```python
from build123d import *

# Parameters (mm, degrees)
ESQUISSE1_R             = 1.5
EXTRUSION1_DEPTH        = 5
ESQUISSE2_W             = 45
ESQUISSE2_H             = 5
EXTRUSION2_DEPTH        = 95
EXTRUSION3_DEPTH        = 5
ESQUISSE4_W             = 95
ESQUISSE4_H             = 50
EXTRUSION4_DEPTH        = 5
ESQUISSE5_W             = 100
ESQUISSE5_H             = 5
EXTRUSION5_DEPTH        = 40
ESQUISSE6_W             = 40
ESQUISSE6_H             = 50
EXTRUSION6_DEPTH        = 5
EXTRUSION7_DEPTH        = 5
ENL_V_MAT_EXTRU_1_REACH = 102
ESQUISSE8_R             = 1.5
ENL_V_MAT_EXTRU_2_REACH = 7
ESQUISSE9_R             = 1.5
BOSS_EXTRU_1_DEPTH      = 5
BOSS_EXTRU_2_DEPTH      = 5
ESQUISSE16_R            = 1.5
ENL_V_MAT_EXTRU_3_DEPTH = 4


with BuildPart() as part:
    # Esquisse1 → Extrusion1 (new body)
    with BuildSketch(Plane.XY):
        Polygon((0, 0), (45, 0), (45, 45), (45, 55), (0, 55), (0, 45), align=None)
        with Locations((31.692388155, 31.692388155)):
            Circle(ESQUISSE1_R, mode=Mode.SUBTRACT)
        with Locations((31.692388155, 13.307611845)):
            Circle(ESQUISSE1_R, mode=Mode.SUBTRACT)
        with Locations((13.307611845, 13.307611845)):
            Circle(ESQUISSE1_R, mode=Mode.SUBTRACT)
        with Locations((13.307611845, 31.692388155)):
            Circle(ESQUISSE1_R, mode=Mode.SUBTRACT)
        with BuildLine():
            Line((13.5, 26.858898944), (13.5, 18.141101056))
            ThreePointArc((13.5, 18.141101056), (22.5, 12.5), (31.5, 18.141101056))
            Line((31.5, 18.141101056), (31.5, 26.858898944))
            ThreePointArc((31.5, 26.858898944), (22.5, 32.5), (13.5, 26.858898944))
        make_face(mode=Mode.SUBTRACT)
    extrude(amount=EXTRUSION1_DEPTH)

    # Esquisse2 → Extrusion2 (add)
    with BuildSketch(Plane.XY.offset(5)):
        with Locations((22.5, 2.5)):
            Rectangle(ESQUISSE2_W, ESQUISSE2_H)
    extrude(amount=EXTRUSION2_DEPTH)

    # Esquisse3 → Extrusion3 (add)
    with BuildSketch(Plane(origin=(45, 0, 0), x_dir=(0, 0, -1), z_dir=(1, 0, 0))):
        Polygon((-5, 5), (-5, 55), (-25, 55), (-25, 50), (-55, 5), align=None)
    extrude(amount=-EXTRUSION3_DEPTH)

    # Esquisse4 → Extrusion4 (add)
    with BuildSketch(Plane.ZY):
        with Locations((52.5, 30)):
            Rectangle(ESQUISSE4_W, ESQUISSE4_H)
    extrude(amount=-EXTRUSION4_DEPTH)

    # Esquisse5 → Extrusion5 (add)
    with BuildSketch(Plane.ZY):
        with Locations((50, 2.5)):
            Rectangle(ESQUISSE5_W, ESQUISSE5_H)
    extrude(amount=EXTRUSION5_DEPTH)

    # Esquisse6 → Extrusion6 (add)
    with BuildSketch(Plane.XY.offset(100)):
        with Locations((-20, 30)):
            Rectangle(ESQUISSE6_W, ESQUISSE6_H)
    extrude(amount=-EXTRUSION6_DEPTH)

    # Esquisse7 → Extrusion7 (add)
    with BuildSketch(Plane.ZY.offset(40)):
        Polygon((95, 5), (95, 55), (75, 55), (75, 50), (45, 5), align=None)
    extrude(amount=-EXTRUSION7_DEPTH)

    # Esquisse8 → Enlèv. mat.-Extru.1 (cut, up to next)
    with BuildSketch(Plane.XY.offset(100), mode=Mode.PRIVATE) as enl_v_mat_extru_1_sk1:
        with Locations((-8.307611845, 13.307611845)):
            Circle(ESQUISSE8_R)
    enl_v_mat_extru_1_tool1 = extrude(enl_v_mat_extru_1_sk1.sketch, amount=-ENL_V_MAT_EXTRU_1_REACH, mode=Mode.PRIVATE) & part.part
    add(enl_v_mat_extru_1_tool1.solids().sort_by_distance((-8.307612, 13.307612, 100))[0], mode=Mode.SUBTRACT)
    # Esquisse8 → Enlèv. mat.-Extru.1 (cut, up to next)
    with BuildSketch(Plane.XY.offset(100), mode=Mode.PRIVATE) as enl_v_mat_extru_1_sk2:
        with Locations((-8.307611845, 31.692388155)):
            Circle(ESQUISSE8_R)
    enl_v_mat_extru_1_tool2 = extrude(enl_v_mat_extru_1_sk2.sketch, amount=-ENL_V_MAT_EXTRU_1_REACH, mode=Mode.PRIVATE) & part.part
    add(enl_v_mat_extru_1_tool2.solids().sort_by_distance((-8.307612, 31.692388, 100))[0], mode=Mode.SUBTRACT)
    # Esquisse8 → Enlèv. mat.-Extru.1 (cut, up to next)
    with BuildSketch(Plane.XY.offset(100), mode=Mode.PRIVATE) as enl_v_mat_extru_1_sk3:
        with Locations((-26.692388155, 31.692388155)):
            Circle(ESQUISSE8_R)
    enl_v_mat_extru_1_tool3 = extrude(enl_v_mat_extru_1_sk3.sketch, amount=-ENL_V_MAT_EXTRU_1_REACH, mode=Mode.PRIVATE) & part.part
    add(enl_v_mat_extru_1_tool3.solids().sort_by_distance((-26.692388, 31.692388, 100))[0], mode=Mode.SUBTRACT)
    # Esquisse8 → Enlèv. mat.-Extru.1 (cut, up to next)
    with BuildSketch(Plane.XY.offset(100), mode=Mode.PRIVATE) as enl_v_mat_extru_1_sk4:
        with Locations((-26.692388155, 13.307611845)):
            Circle(ESQUISSE8_R)
    enl_v_mat_extru_1_tool4 = extrude(enl_v_mat_extru_1_sk4.sketch, amount=-ENL_V_MAT_EXTRU_1_REACH, mode=Mode.PRIVATE) & part.part
    add(enl_v_mat_extru_1_tool4.solids().sort_by_distance((-26.692388, 13.307612, 100))[0], mode=Mode.SUBTRACT)
    # Esquisse8 → Enlèv. mat.-Extru.1 (cut, up to next)
    with BuildSketch(Plane.XY.offset(100), mode=Mode.PRIVATE) as enl_v_mat_extru_1_sk5:
        with BuildLine():
            Line((-26.5, 18.141101056), (-26.5, 26.858898944))
            ThreePointArc((-26.5, 26.858898944), (-17.5, 32.5), (-8.5, 26.858898944))
            Line((-8.5, 26.858898944), (-8.5, 18.141101056))
            ThreePointArc((-8.5, 18.141101056), (-17.5, 12.5), (-26.5, 18.141101056))
        make_face()
    enl_v_mat_extru_1_tool5 = extrude(enl_v_mat_extru_1_sk5.sketch, amount=-ENL_V_MAT_EXTRU_1_REACH, mode=Mode.PRIVATE) & part.part
    add(enl_v_mat_extru_1_tool5.solids().sort_by_distance((-17.5, 22.5, 100))[0], mode=Mode.SUBTRACT)

    # Esquisse9 → Enlèv. mat.-Extru.2 (cut, up to next)
    with BuildSketch(Plane(origin=(0, 5, 0), x_dir=(-1, 0, 0), z_dir=(0, 1, 0)), mode=Mode.PRIVATE) as enl_v_mat_extru_2_sk1:
        with Locations((-40, 95)):
            Circle(ESQUISSE9_R)
    enl_v_mat_extru_2_tool1 = extrude(enl_v_mat_extru_2_sk1.sketch, amount=-ENL_V_MAT_EXTRU_2_REACH, mode=Mode.PRIVATE) & part.part
    add(enl_v_mat_extru_2_tool1.solids().sort_by_distance((40, 5, 95))[0], mode=Mode.SUBTRACT)
    # Esquisse9 → Enlèv. mat.-Extru.2 (cut, up to next)
    with BuildSketch(Plane(origin=(0, 5, 0), x_dir=(-1, 0, 0), z_dir=(0, 1, 0)), mode=Mode.PRIVATE) as enl_v_mat_extru_2_sk2:
        with Locations((-10, 95)):
            Circle(ESQUISSE9_R)
    enl_v_mat_extru_2_tool2 = extrude(enl_v_mat_extru_2_sk2.sketch, amount=-ENL_V_MAT_EXTRU_2_REACH, mode=Mode.PRIVATE) & part.part
    add(enl_v_mat_extru_2_tool2.solids().sort_by_distance((10, 5, 95))[0], mode=Mode.SUBTRACT)
    # Esquisse9 → Enlèv. mat.-Extru.2 (cut, up to next)
    with BuildSketch(Plane(origin=(0, 5, 0), x_dir=(-1, 0, 0), z_dir=(0, 1, 0)), mode=Mode.PRIVATE) as enl_v_mat_extru_2_sk3:
        with Locations((35, 5)):
            Circle(ESQUISSE9_R)
    enl_v_mat_extru_2_tool3 = extrude(enl_v_mat_extru_2_sk3.sketch, amount=-ENL_V_MAT_EXTRU_2_REACH, mode=Mode.PRIVATE) & part.part
    add(enl_v_mat_extru_2_tool3.solids().sort_by_distance((-35, 5, 5))[0], mode=Mode.SUBTRACT)
    # Esquisse9 → Enlèv. mat.-Extru.2 (cut, up to next)
    with BuildSketch(Plane(origin=(0, 5, 0), x_dir=(-1, 0, 0), z_dir=(0, 1, 0)), mode=Mode.PRIVATE) as enl_v_mat_extru_2_sk4:
        with Locations((5, 5)):
            Circle(ESQUISSE9_R)
    enl_v_mat_extru_2_tool4 = extrude(enl_v_mat_extru_2_sk4.sketch, amount=-ENL_V_MAT_EXTRU_2_REACH, mode=Mode.PRIVATE) & part.part
    add(enl_v_mat_extru_2_tool4.solids().sort_by_distance((-5, 5, 5))[0], mode=Mode.SUBTRACT)
    # Esquisse9 → Enlèv. mat.-Extru.2 (cut, up to next)
    with BuildSketch(Plane(origin=(0, 5, 0), x_dir=(-1, 0, 0), z_dir=(0, 1, 0)), mode=Mode.PRIVATE) as enl_v_mat_extru_2_sk5:
        with Locations((-40, 60)):
            Circle(ESQUISSE9_R)
    enl_v_mat_extru_2_tool5 = extrude(enl_v_mat_extru_2_sk5.sketch, amount=-ENL_V_MAT_EXTRU_2_REACH, mode=Mode.PRIVATE) & part.part
    add(enl_v_mat_extru_2_tool5.solids().sort_by_distance((40, 5, 60))[0], mode=Mode.SUBTRACT)
    # Esquisse9 → Enlèv. mat.-Extru.2 (cut, up to next)
    with BuildSketch(Plane(origin=(0, 5, 0), x_dir=(-1, 0, 0), z_dir=(0, 1, 0)), mode=Mode.PRIVATE) as enl_v_mat_extru_2_sk6:
        with Locations((35, 40)):
            Circle(ESQUISSE9_R)
    enl_v_mat_extru_2_tool6 = extrude(enl_v_mat_extru_2_sk6.sketch, amount=-ENL_V_MAT_EXTRU_2_REACH, mode=Mode.PRIVATE) & part.part
    add(enl_v_mat_extru_2_tool6.solids().sort_by_distance((-35, 5, 40))[0], mode=Mode.SUBTRACT)

    # Esquisse11 → Boss.-Extru.1 (add)
    with BuildSketch(Plane(origin=(0, 55, 0), x_dir=(1, 0, 0), z_dir=(0, 1, 0))):
        Polygon((22.5, -5), (5, -25), (5, 0), (40, 0), (40, -25), align=None)
    extrude(amount=-BOSS_EXTRU_1_DEPTH)

    # Esquisse12 → Boss.-Extru.2 (add)
    with BuildSketch(Plane(origin=(0, 55, 0), x_dir=(1, 0, 0), z_dir=(0, 1, 0))):
        Polygon((0, -75), (-17.5, -95), (-35, -75), (-35, -100), (0, -100), align=None)
    extrude(amount=-BOSS_EXTRU_2_DEPTH)

    # Esquisse16 → Enlèv. mat.-Extru.3 (cut)
    with BuildSketch(Plane(origin=(0, 55, 0), x_dir=(1, 0, 0), z_dir=(0, 1, 0))):
        with Locations((-5, -90)):
            Circle(ESQUISSE16_R)
        with Locations((-30, -90)):
            Circle(ESQUISSE16_R)
        with Locations((10, -10)):
            Circle(ESQUISSE16_R)
        with Locations((35, -10)):
            Circle(ESQUISSE16_R)
    extrude(amount=-ENL_V_MAT_EXTRU_3_DEPTH, mode=Mode.SUBTRACT)


solid = part.part
```
Read the model definition and answer for the solid it produces. Units are mm, in the model's axes. A direction names the side the tool comes from. Give positions to 0.01 mm unless a question says otherwise; leave off trailing zeros. Write each loop counter-clockwise with the first axis right and the second up, starting at its lowest first coordinate (ties: lowest second). Pieces come first, ordered by that corner, then holes. Notation, with made-up numbers: (-13.75, -14) -> (1.25, -14) arc R18 ccw to (1.25, 0) -> close; hole circle Ø8 at (72, 0.25). An arc over 180 degrees is marked (long way). Answer in a Markdown table with one row per item.
1) Section B-B on z = 40 is taken. Give the vertices of the cut face in (x, y).
Results list:
| item | result |
|---|---|
| outline | (-40, 0) -> (-36.5, 0) -> (-36.5, 5) -> (-40, 5) -> close; (-33.5, 0) -> (45, 0) -> (45, 27.5) -> (40, 27.5) -> (40, 5) -> (5, 5) -> (5, 55) -> (0, 55) -> (0, 5) -> (-33.5, 5) -> close |
2) Section D-D on z = 78 is taken. Give the vertices of the cut face in (x, y) (3 decimals).
Results list:
| item | result |
|---|---|
| outline | (-40, 0) -> (45, 0) -> (45, 5) -> (5, 5) -> (5, 55) -> (-2.625, 55) -> (-2.625, 50) -> (0, 50) -> (0, 5) -> (-35, 5) -> (-35, 50) -> (-32.375, 50) -> (-32.375, 55) -> (-40, 55) -> close |
3) Section C-C on x = -5 is taken. Give the vertices of the cut face in (y, z).
Results list:
| item | result |
|---|---|
| outline | (0, 0) -> (5, 0) -> (5, 3.5) -> (0, 3.5) -> close; (0, 6.5) -> (5, 6.5) -> (5, 95) -> (50, 95) -> (50, 80.71) -> (55, 80.71) -> (55, 88.5) -> (51, 88.5) -> (51, 91.5) -> (55, 91.5) -> (55, 100) -> (0, 100) -> close |
4) Each of these flat-tipped pins is pushed along its axis until it touches: pin 1 Ø4 at (y, z) = (24.5, 2) entering from -X; pin 2 Ø1 at (x, y) = (-25, 32) entering from -Z; pin 3 Ø1 at (y, z) = (11.5, 54.5) entering from +X. Where does it stop, or does it pass through?
Results list:
| item | result |
|---|---|
| pin 1 | x = 0 |
| pin 2 | z = 95 |
| pin 3 | x = 5 |
5) Section A-A on y = 23 is taken. Give the vertices of the cut face in (x, z).
Results list:
| item | result |
|---|---|
| outline | (-40, 57) -> (-35, 57) -> (-35, 95) -> (-26.5, 95) -> (-26.5, 100) -> (-40, 100) -> close; (-8.5, 95) -> (0, 95) -> (0, 0) -> (13.5, 0) -> (13.5, 5) -> (5, 5) -> (5, 100) -> (-8.5, 100) -> close; (31.5, 0) -> (45, 0) -> (45, 43) -> (40, 43) -> (40, 5) -> (31.5, 5) -> close |
6) A tool of negligible diameter and unlimited length cuts with its end or side. For faces 4 (the flat face through (-37.5, 27.8, 60.2)), 5 (the flat face through (35, 51, 10)), 6 (the flat face through (5, 30, 52)), from which of +Z, -Z, +X, -X, +Y, -Y can it reach the whole face along a straight path? Write none if from no direction.
Results list:
| item | result |
|---|---|
| face 4 | -Z, -X, +Y |
| face 5 | +Y |
| face 6 | +Z |
7) Straight lines are drawn through the part: line 1 (X direction, y = 3.35, z = 95); line 2 (X direction, y = 22, z = 15.5); line 3 (Z direction, x = -5, y = 2.35). For each, find the intervals that lie inside material, in ascending order. Write a range as [from, to].
Results list:
| item | result |
|---|---|
| line 1 | [-40, 8.5], [11.5, 38.5], [41.5, 45] |
| line 2 | [0, 5], [40, 45] |
| line 3 | [0, 3.5], [6.5, 100] |
8) Determine the mould class of faces 1 (the flat face through (31.37, 52.54, 15.14)), 2 (the flat face through (-30, 51, 90)), 3 (the flat face through (40, 23, 25)) for opening direction Z: released by +Z, released by -Z, zero draft, split by the parting line, or undercut.
Results list:
| item | result |
|---|---|
| face 1 | released by +Z |
| face 2 | undercut |
| face 3 | zero draft |
